Here's how the part is built. I have some questions about the finished solid (model axes, mm). Face numbers are marked on the shaded views. Round coordinates to 2 decimals unless told otherwise and drop trailing zeros. Write each loop counter-clockwise with the first axis right and the second up, starting at its lowest first coordinate (ties: lowest second). Pieces come first, ordered by that corner, then holes. Notation, with made-up numbers: (-22, 72) -> (-2, 72) arc R20 ccw to (-2, 90) -> close; hole circle Ø8 at (50, 67.5). An arc over 180 degrees is marked (long way). Answer in a Markdown table with one row per item.
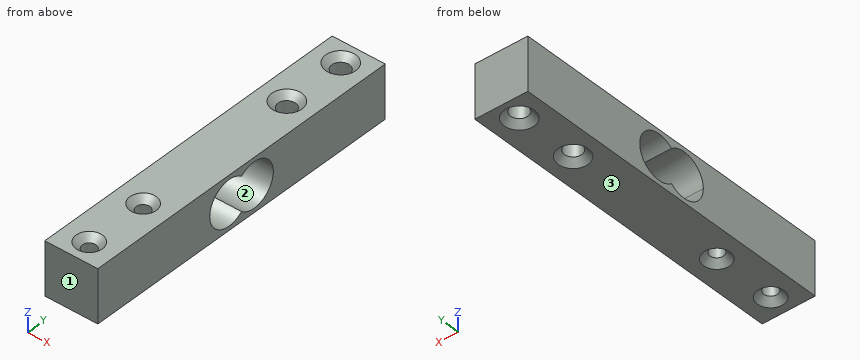
from build123d import *

# Parameters (mm, degrees)
F0_W     = 12.7
F0_H     = 80
F0_R     = 1.65
F0_R_2   = 2.1
F1_DEPTH = 12.7
F3_DEPTH = 12.701
F4_SIZE  = 1.5
F5_SIZE  = 1.5


with BuildPart() as f1:
    # F0 (on Top) → F1 (new body)
    with BuildSketch(Plane.XY):
        Rectangle(F0_W, F0_H)
        with Locations((0, -35)):
            Circle(F0_R, mode=Mode.SUBTRACT)
        with Locations((0, -20)):
            Circle(F0_R, mode=Mode.SUBTRACT)
        with Locations((0, 20)):
            Circle(F0_R_2, mode=Mode.SUBTRACT)
        with Locations((0, 35)):
            Circle(F0_R_2, mode=Mode.SUBTRACT)
    extrude(amount=F1_DEPTH)

    # F2 (on face) → F3 (cut, through all)
    with BuildSketch(Plane(origin=(-6.35, 0, 0), x_dir=(0, -1, 0), z_dir=(-1, 0, 0))):
        with BuildLine():
            ThreePointArc((0, 2.303705), (-1.85, 6.35), (0, 10.396295))
            ThreePointArc((0, 10.396295), (-8.85, 6.35), (0, 2.303705))
        make_face()
        with BuildLine():
            ThreePointArc((0, 10.396295), (1.365568, 8.574579), (1.85, 6.35))
            ThreePointArc((1.85, 6.35), (1.365568, 4.125421), (0, 2.303705))
            ThreePointArc((0, 2.303705), (5.724579, 1.484432), (8.85, 6.35))
            ThreePointArc((8.85, 6.35), (5.724579, 11.215568), (0, 10.396295))
        make_face()
        with BuildLine():
            ThreePointArc((0, 2.303705), (1.365568, 4.125421), (1.85, 6.35))
            ThreePointArc((1.85, 6.35), (1.365568, 8.574579), (0, 10.396295))
            ThreePointArc((0, 10.396295), (-1.85, 6.35), (0, 2.303705))
        make_face()
    extrude(amount=-F3_DEPTH, mode=Mode.SUBTRACT)

    # F4
    f4_edges = [f1.edges().sort_by_distance(p)[0] for p in [
        (-2.1, 35, 12.7),
        (-2.1, 20, 12.7),
        (-1.65, -20, 12.7),
        (-1.65, -35, 12.7),
    ]]
    chamfer(f4_edges, length=F4_SIZE)

    # F5
    f5_edges = [f1.edges().sort_by_distance(p)[0] for p in [
        (-2.1, 35, 0),
        (-2.1, 20, 0),
        (-1.65, -20, 0),
        (-1.65, -35, 0),
    ]]
    chamfer(f5_edges, length=F5_SIZE)


solid = f1.part
1) I need wall thicknesses on line 1 (Z direction, x = 3.25, y = 3.5); line 2 (Y direction, x = 0, z = 9); line 3 (Y direction, x = 1, z = 4.75). Which ranges of each line are inside material? Lowest first, please. Write a range as [from, to].
Response:
| item | result |
|---|---|
| line 1 | z = [0, 1], [11.7, 12.7] |
| line 2 | y = [-40, -36.65], [-33.35, -21.65], [-18.35, -8.15], [8.15, 17.9], [22.1, 32.9], [37.1, 40] |
| line 3 | y = [-40, -36.31], [-33.69, -21.31], [-18.69, -8.61], [8.61, 18.15], [21.85, 33.15], [36.85, 40] |
2) For pin 1 (2 mm diameter, centred on x = 0, y = -35, fed in from +Z); pin 2 (1.5 mm diameter, centred on x = -1.5, y = 20, fed in from -Z), each with a flat end and sliding along its axis, tell me the tip position at first contact or that it passes through.
Response:
| item | result |
|---|---|
| pin 1 | passes through |
| pin 2 | stops at z = 1.35 |
3) I want a section at D-D, the plane y = -20. List the corners of the cut face in (x, z) for me, and give its area (3 significant figures).
Response:
| item | result |
|---|---|
| outline | (-6.35, 0) -> (-3.15, 0) -> (-1.65, 1.5) -> (-1.65, 11.2) -> (-3.15, 12.7) -> (-6.35, 12.7) -> close; (1.65, 1.5) -> (3.15, 0) -> (6.35, 0) -> (6.35, 12.7) -> (3.15, 12.7) -> (1.65, 11.2) -> close |
| area | 115 mm^2 |
4) I want a section at C-C, the plane x = 0.75. Count the separate pieces of the cut face and the enclosed holes in it, and give its area (3 significant figures).
Response:
| item | result |
|---|---|
| separate pieces | 5 |
| enclosed holes | 1 |
| area | 664 mm^2 |
5) I want a section at A-A, the plane y = 3.5. List the corners of the cut face in (x, z) for me, and give its area (3 significant figures).
Response:
| item | result |
|---|---|
| outline | (-6.35, 0) -> (6.35, 0) -> (6.35, 1) -> (-6.35, 1) -> close; (-6.35, 11.7) -> (6.35, 11.7) -> (6.35, 12.7) -> (-6.35, 12.7) -> close |
| area | 25.4 mm^2 |
6) I want a section at B-B, the plane z = 5.5. List the corners of the cut face in (x, y) for me.
Response:
| item | result |
|---|---|
| outline | (-6.35, -40) -> (6.35, -40) -> (6.35, -8.78) -> (-6.35, -8.78) -> close; (-6.35, 8.78) -> (6.35, 8.78) -> (6.35, 40) -> (-6.35, 40) -> close; hole circle Ø4.2 at (0, 20); hole circle Ø4.2 at (0, 35); hole circle Ø3.3 at (0, -35); hole circle Ø3.3 at (0, -20) |
7) We'd pull the mould along Y, two halves only. Please class the marked faces 1, 2 and 3: +Y half, -Y half, draft (parallel to the pull), parting line (faces both ways), or undercut.
Response:
| item | result |
|---|---|
| face 1 | -Y half |
| face 2 | undercut |
| face 3 | draft |
